from build123d import *

# Parameters (mm, degrees)
SKETCH1_W           = 400
SKETCH1_H           = 398
SKETCH1_R           = 2.5
BOSS_EXTRUDE1_DEPTH = 2
SKETCH2_R           = 15
BOSS_EXTRUDE2_DEPTH = 8


with BuildPart() as part:
    # Sketch1 → Boss-Extrude1 (new body)
    with BuildSketch(Plane(origin=(0, 0, 0), x_dir=(1, 0, 0), z_dir=(0, 1, 0))):
        with Locations((200, 199)):
            Rectangle(SKETCH1_W, SKETCH1_H)
        with Locations(Location((50, 15, 0), (0, 0, 270))):
            Circle(SKETCH1_R, mode=Mode.SUBTRACT)
        with Locations(Location((200, 15, 0), (0, 0, 270))):
            Circle(SKETCH1_R, mode=Mode.SUBTRACT)
        with Locations(Location((350, 15, 0), (0, 0, 270))):
            Circle(SKETCH1_R, mode=Mode.SUBTRACT)
        with Locations(Location((350, 383, 0), (0, 0, 90))):
            Circle(SKETCH1_R, mode=Mode.SUBTRACT)
        with Locations(Location((200, 383, 0), (0, 0, 90))):
            Circle(SKETCH1_R, mode=Mode.SUBTRACT)
        with Locations(Location((50, 383, 0), (0, 0, 90))):
            Circle(SKETCH1_R, mode=Mode.SUBTRACT)
    extrude(amount=BOSS_EXTRUDE1_DEPTH)

    # Sketch2 → Boss-Extrude2 (add)
    with BuildSketch(Plane.XZ):
        with Locations(Location((18, -18, 0), (0, 0, 270))):
            Circle(SKETCH2_R)
        with Locations(Location((382, -18, 0), (0, 0, 90))):
            Circle(SKETCH2_R)
        with Locations(Location((382, -380, 0), (0, 0, 270))):
            Circle(SKETCH2_R)
        with Locations(Location((18, -380, 0), (0, 0, 90))):
            Circle(SKETCH2_R)
    extrude(amount=BOSS_EXTRUDE2_DEPTH)


solid = part.part
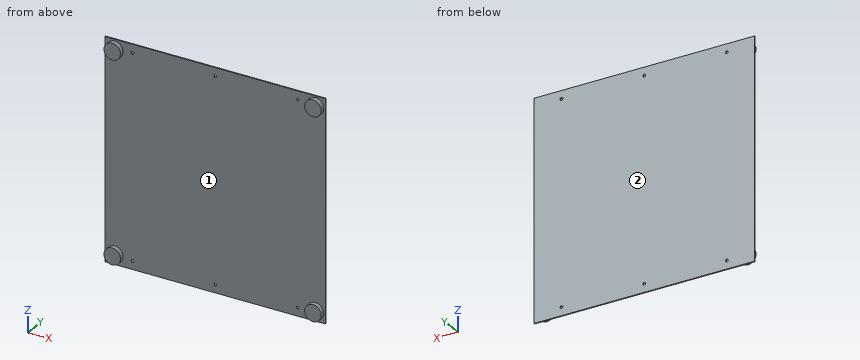
Input: part model. Units: mm. Frame: model coordinates. Face numbers are marked on the shaded views. A direction names the side the tool comes from. Coordinates: 2 decimals unless noted, no trailing zeros. Write each loop counter-clockwise with the first axis right and the second up, starting at its lowest first coordinate (ties: lowest second). Pieces come first, ordered by that corner, then holes. Notation, with made-up numbers: M -1.75,58 L 21.25,58 A14 ccw 21.25,75 Z; hole C 1,37.5 d11. An arc over 180 degrees is marked long. Answer as a JSON object with one key per item and string values. Group by question number.
(1) Ray query, line 1 along Z through (x, y) = (200, 1.25); line 2 along X through (y, z) = (1.45, -383); line 3 along Y through (x, z) = (42.5, -366.5). Return the intervals inside material, ascending. Write a range as [from, to].
(2) Set-up query: the marked faces 1 and 2. Return all of +Z, -Z, +X, -X, +Y, -Y with unobstructed straight access to the full face (end or side cutting, diameter ignored); none if empty.
(3) Contact query for flat-ended pins moving along their axis: P1, Ø1.5, axis at x = 330, y = 1, coming from the +Z side; P2, Ø6.5, axis at x = 350, z = -383, coming from the -Y side. Output: stop coordinate, or through.
(4) Section C-C on z = -372.5. Output: boundary loops of the cut face in (x, y), plus the area to 3 significant figures.
(5) Section D-D on x = 103. Output: boundary loops of the cut face in (y, z).
(6) Section B-B on x = 382. Output: boundary loops of the cut face in (y, z).
(7) Section A-A on y = -6. Output: boundary loops of the cut face in (x, z), plus the area to 3 significant figures.
Result set:
{
 "1": {"line 1": "z = [-398, -385.5], [-380.5, -17.5], [-12.5, 0]", "line 2": "x = [0, 47.5], [52.5, 197.5], [202.5, 347.5], [352.5, 400]", "line 3": "y = [0, 2]"},
 "2": {"face 1": "-Y", "face 2": "+Z, -Z, +X, -X, +Y"},
 "3": {"P1": "stops at z = 0", "P2": "stops at y = 0"},
 "4": {"outline": "M 0,0 L 5.01,0 L 5.01,-8 L 30.99,-8 L 30.99,0 L 369.01,0 L 369.01,-8 L 394.99,-8 L 394.99,0 L 400,0 L 400,2 L 0,2 Z", "area": "1,220 mm2"},
 "5": {"outline": "M 0,-398 L 2,-398 L 2,0 L 0,0 Z"},
 "6": {"outline": "M -8,-395 L 0,-395 L 0,-398 L 2,-398 L 2,0 L 0,0 L 0,-3 L -8,-3 L -8,-33 L 0,-33 L 0,-365 L -8,-365 Z"},
 "7": {"outline": "C 18,-380 d30; C 18,-18 d30; C 382,-380 d30; C 382,-18 d30", "area": "2,830 mm2"}
}
